Geometry check sheet. Reference: the model listing, model coordinates, mm. A direction names the side the tool comes from. Coordinates: 2 decimals unless noted, no trailing zeros. Order: outer loops, then holes, each group sorted by start corner. A loop starts at its lowest first (then second) coordinate and runs counter-clockwise, first axis right, second up. Notation, with made-up numbers: (-24, -30) - (-13, -30) arc R29 cw to (-13, 9) - close; hole circle Ø7 at (37, 30). An arc over 180 degrees is marked (long way). Return JSON: item names as keys, results as strings. Group by question number.
Item 1: Section check D-D on z = 23.5. Enter the section's corners in (x, y), then the cut area to 3 significant figures.
Item 2: Draft check along X on faces 1 (the flat face through (24.9, 2, 0)), 2 (the cylindrical face through (14.643, 1.972, 26.184)), 3 (the flat face through (-11.87, 1.97, 24.76)), 4 (the cylindrical face through (-30, 2, 0)). Enter one of: pulls with the +X half, pulls with the -X half, needs draft (parallel to the pull), parting line crosses it, or undercut.
Item 3: Gauge pin test, flat ends, axial feed: pin 1 (10 mm diameter, centred on x = 7, z = -21.5, fed in from -Y); pin 2 (1 mm diameter, centred on x = 6, y = 1, fed in from -Z). Record the tip position at first contact, or that the pin passes through.
Item 4: Section check C-C on x = -11.5. Enter the section's corners in (y, z), then the cut area to 3 significant figures.
Item 5: Scan lines: probe 1 along Z at (x, y) = (-11, 2.45); probe 2 along Z at (x, y) = (-13, 0.55); probe 3 along Z at (x, y) = (0.5, 1.85). Record each from-to range of solid material in increasing order.
Item 6: Section check B-B on y = 1.3. Enter the section's corners in (x, z).
Item 7: Tool access check on faces 5 (the flat face through (-15.508, 1.972, -22.66)), 6 (the flat face through (-11.87, 1.97, -24.76)), 7 (the flat face through (-15.508, 1.972, 22.66)). Record the directions out of +Z, -Z, +X, -X, +Y, -Y that give a thin tool (end or side, any length) a straight path to the whole face; none if there is none.
Item 8: Section check A-A on x = 26. Enter the section's corners in (y, z), then the cut area to 3 significant figures.
from build123d import *

# Parameters (mm, degrees)
CROQUIS1_R              = 30
SALIENTE_EXTRUIR1_DEPTH = 4
CORTAR_EXTRUIR2_REACH   = 44.615
CROQUIS2_W              = 10.2
CROQUIS2_H              = 4.2
MATRIZC1_COUNT          = 3


with BuildPart() as part:
    # Croquis1 → Saliente-Extruir1 (new body)
    with BuildSketch(Plane(origin=(0, 0, 0), x_dir=(1, 0, 0), z_dir=(0, 1, 0))):
        with Locations(Location((0, 0, 0), (0, 0, 270))):
            Circle(CROQUIS1_R)
    extrude(amount=SALIENTE_EXTRUIR1_DEPTH)

    # Croquis2 → Cortar-Extruir2 (cut, up to next)
    with BuildSketch(Plane(origin=(0, 0, 0), x_dir=(1, 0, 0), z_dir=(0, 1, 0)), mode=Mode.PRIVATE) as cortar_extruir2_sk1:
        with Locations((30, 0)):
            Rectangle(CROQUIS2_W, CROQUIS2_H)
    cortar_extruir2_tool1 = extrude(cortar_extruir2_sk1.sketch, amount=CORTAR_EXTRUIR2_REACH, mode=Mode.PRIVATE) & part.part
    cortar_extruir2 = cortar_extruir2_tool1.solids().sort_by_distance((30, 0, 0))[0]
    add(cortar_extruir2, mode=Mode.SUBTRACT)

    # MatrizC1: Cortar-Extruir2 ×3 about axis
    matrizc1_axis = Axis((0, 0, 0), (0, 1, 0))
    for i in range(1, MATRIZC1_COUNT):
        add(cortar_extruir2.rotate(matrizc1_axis, i * 360 / MATRIZC1_COUNT), mode=Mode.SUBTRACT)


solid = part.part
Computed:
{
 "1": {"outline": "(-18.65, 0) - (-15.99, 0) - (-15.99, 4) - (-18.65, 4) - close; (-11.14, 0) - (18.65, 0) - (18.65, 4) - (-11.14, 4) - close", "area": "130 mm²"},
 "2": {"face 1": "pulls with the +X half", "face 2": "parting line crosses it", "face 3": "undercut", "face 4": "pulls with the -X half"},
 "3": {"pin 1": "stops at y = 0", "pin 2": "stops at z = -29.49"},
 "4": {"outline": "(0, -27.71) - (4, -27.71) - (4, -24.12) - (0, -24.12) - close; (0, -22.11) - (4, -22.11) - (4, 22.11) - (0, 22.11) - close; (0, 24.12) - (4, 24.12) - (4, 27.71) - (0, 27.71) - close", "area": "206 mm²"},
 "5": {"probe 1": "z = -27.91 to -23.25, -22.4 to 22.4, 23.25 to 27.91", "probe 2": "z = -27.04 to -26.72, -21.25 to 21.25, 26.72 to 27.04", "probe 3": "z = -30 to 30"},
 "6": {"outline": "(-16.78, -24.87) - (-14.27, -20.51) - (-10.63, -22.61) - (-13.14, -26.97) arc R30 ccw to (29.93, -2.1) - (24.9, -2.1) - (24.9, 2.1) - (29.93, 2.1) arc R30 ccw to (-13.14, 26.97) - (-10.63, 22.61) - (-14.27, 20.51) - (-16.78, 24.87) arc R30 ccw to start"},
 "7": {"face 5": "-Z, +Y, -Y", "face 6": "+Y, -Y", "face 7": "+Z, +Y, -Y"},
 "8": {"outline": "(0, -14.97) - (4, -14.97) - (4, -2.1) - (0, -2.1) - close; (0, 2.1) - (4, 2.1) - (4, 14.97) - (0, 14.97) - close", "area": "103 mm²"}
}
